Can you work these out from the model? Positions are in its coordinate system, mm. A direction names the side the tool comes from. Round coordinates to 2 decimals unless told otherwise and drop trailing zeros. Loops run counter-clockwise (first coordinate to the right, second up) from the corner with the lowest first, then second, coordinate; pieces in that order, holes last. Notation, with made-up numbers: (79, -32) -> (96, -32) arc R32 ccw to (96, -3) -> close; hole circle Ø2 at (52.25, 22.5). An arc over 180 degrees is marked (long way). Use a Markdown table: item, result.
from build123d import *

# Parameters (mm, degrees)
F1_DEPTH = 127
F2_R     = 1.3462
F3_DEPTH = 25.2994
F5_DEPTH = 25.2994


with BuildPart() as f1:
    # F0 (on Right) → F1 (new body)
    with BuildSketch(Plane.YZ):
        with BuildLine():
            Line((-10.285505, -7.297242), (-10.285505, -8.262442))
            Line((-10.285505, -8.262442), (15.012895, -8.262442))
            Line((15.012895, -8.262442), (15.012895, 4.335958))
            Line((15.012895, 4.335958), (14.047695, 4.335958))
            ThreePointArc((14.047695, 4.335958), (12.521052, 3.703602), (11.888695, 2.176958))
            Line((11.888695, 2.176958), (11.888695, -2.979242))
            ThreePointArc((11.888695, -2.979242), (11.256339, -4.505885), (9.729695, -5.138242))
            Line((9.729695, -5.138242), (-8.126505, -5.138242))
            ThreePointArc((-8.126505, -5.138242), (-9.653148, -5.770598), (-10.285505, -7.297242))
        make_face()
    extrude(amount=F1_DEPTH)

    # F2 (on face) → F3 (cut, through all)
    with BuildSketch(Plane(origin=(0, 15.012895, 0), x_dir=(-1, 0, 0), z_dir=(0, 1, 0))):
        with Locations((-31.75, -2.166442)):
            Circle(F2_R)
        with Locations((-95.25, -2.166442)):
            Circle(F2_R)
    extrude(amount=-F3_DEPTH, mode=Mode.SUBTRACT)

    # F4 (on face) → F5 (cut, through all)
    with BuildSketch(Plane(origin=(0, 15.012895, 0), x_dir=(-1, 0, 0), z_dir=(0, 1, 0))):
        with BuildLine():
            Line((-108.6612, -1.277442), (-108.6612, 4.335958))
            Line((-108.6612, 4.335958), (-118.8212, 4.335958))
            Line((-118.8212, 4.335958), (-118.8212, -1.277442))
            ThreePointArc((-118.8212, -1.277442), (-118.449226, -2.175467), (-117.5512, -2.547442))
            Line((-117.5512, -2.547442), (-109.9312, -2.547442))
            ThreePointArc((-109.9312, -2.547442), (-109.033174, -2.175467), (-108.6612, -1.277442))
        make_face()
        with BuildLine():
            Line((-47.7012, -3.182442), (-47.7012, 4.335958))
            Line((-47.7012, 4.335958), (-60.4012, 4.335958))
            Line((-60.4012, 4.335958), (-60.4012, -3.182442))
            ThreePointArc((-60.4012, -3.182442), (-60.029226, -4.080467), (-59.1312, -4.452442))
            Line((-59.1312, -4.452442), (-48.9712, -4.452442))
            ThreePointArc((-48.9712, -4.452442), (-48.073174, -4.080467), (-47.7012, -3.182442))
        make_face()
    extrude(amount=-F5_DEPTH, mode=Mode.SUBTRACT)


solid = f1.part
1. I want a section at B-B (x = 111.5). Please give me the cut outline in (y, z).
Answer sheet:
| item | result |
|---|---|
| outline | (-10.29, -8.26) -> (15.01, -8.26) -> (15.01, -2.55) -> (11.89, -2.55) -> (11.89, -2.98) arc R2.16 cw to (9.73, -5.14) -> (-8.13, -5.14) arc R2.16 ccw to (-10.29, -7.3) -> close |
2. I want a section at A-A (x = 95.25). Please give me the cut outline in (y, z).
Answer sheet:
| item | result |
|---|---|
| outline | (-10.29, -8.26) -> (15.01, -8.26) -> (15.01, -3.51) -> (11.82, -3.51) arc R2.16 cw to (9.73, -5.14) -> (-8.13, -5.14) arc R2.16 ccw to (-10.29, -7.3) -> close; (11.89, -0.82) -> (15.01, -0.82) -> (15.01, 4.34) -> (14.05, 4.34) arc R2.16 ccw to (11.89, 2.18) -> close |
3. I want a section at C-C (y = -4.25). Please give me the cut outline in (x, z).
Answer sheet:
| item | result |
|---|---|
| outline | (0, -8.26) -> (127, -8.26) -> (127, -5.14) -> (0, -5.14) -> close |
4. I need wall thicknesses on line 1 (Z direction, x = 31.75, y = 14.2); line 2 (X direction, y = 13, z = 3.75); line 3 (Z direction, x = 92, y = -3). Which ranges of each line are inside material? Lowest first, please.
Answer sheet:
| item | result |
|---|---|
| line 1 | z = -8.26 to -3.51, -0.82 to 4.34 |
| line 2 | x = 0 to 47.7, 60.4 to 108.66, 118.82 to 127 |
| line 3 | z = -8.26 to -5.14 |
5. If we mould it in two halves opening along X, with no side actions, what happens to faces 1 (the flat face through (127, 5, -6)), 2 (the cylindrical face through (30.506, 13.44, -2.682)), 3 (the flat face through (63, 1, -5.138))? For each: +X half, -X half, draft (parallel to the pull), parting line (faces both ways), or undercut.
Answer sheet:
| item | result |
|---|---|
| face 1 | +X half |
| face 2 | undercut |
| face 3 | draft |
6. Which directions (+Z, -Z, +X, -X, +Y, -Y) give clear straight access to the entire face, cutting with the end or side of a thin tool? Please do faces 4 (the flat face through (63, 15.013, -2)), 5 (the flat face through (24, 11.889, 0)), 6 (the flat face through (47.701, 13, 1)).
Answer sheet:
| item | result |
|---|---|
| face 4 | +Z, -Z, +X, -X, +Y |
| face 5 | +Z, +X, -X, -Y |
| face 6 | +Z, +Y, -Y |
7. Will these pins go through, and if not, where does the flat tip stop? pin 1 Ø9 at (x, y) = (35.5, -3.5) entering from +Z; pin 2 Ø1.1 at (x, y) = (51.5, 13.5) entering from +Z; pin 3 Ø5.5 at (x, z) = (99.5, -1) entering from -Y.
Answer sheet:
| item | result |
|---|---|
| pin 1 | stops at z = -5.14 |
| pin 2 | stops at z = -4.45 |
| pin 3 | stops at y = 11.75 |
